from build123d import *

# Parameters (mm, degrees)
F1_DEPTH = 7.62
F3_DEPTH = 7.62


with BuildPart() as f1:
    # F0 (on Front) → F1 (new body)
    with BuildSketch(Plane.XZ):
        with BuildLine():
            ThreePointArc((21.0290110962, 0), (21.3248501657, 1.9931047456), (21.4237811773, 4.0056155995))
            ThreePointArc((21.4237811773, 4.0056155995), (-1.1080148506, 24.4259697619), (-19.2200190896, 0))
            ThreePointArc((-19.2200190896, 0), (0.9044960033, -16.5136695746), (21.0290110962, 0))
        make_face()
    extrude(amount=F1_DEPTH)

    # F2 (on Front) → F3 (join)
    with BuildSketch(Plane.XZ):
        with BuildLine():
            ThreePointArc((-16.8698355556, -6.6087017767), (-15.6905339278, -0.7832460117), (-21.5823259205, 0))
            ThreePointArc((-21.5823259205, 0), (-41.5234625412, -12.3382675542), (-47.9722805321, -34.8836556077))
            Line((-47.9722805321, -34.8836556077), (-35.7198044658, -33.9411571622))
            ThreePointArc((-35.7198044658, -33.9411571622), (-31.8794663631, -16.423449292), (-16.8698355556, -6.6087017767))
        make_face()
    extrude(amount=F3_DEPTH)


solid = f1.part
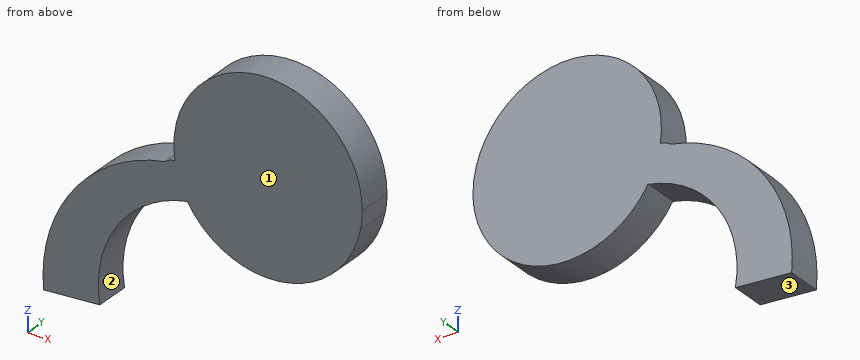
Geometry: final body of the model. Coordinates: model frame, mm. Face numbers are marked on the shaded views. Give positions to 0.01 mm unless a question says otherwise; leave off trailing zeros. Loops run counter-clockwise (first coordinate to the right, second up) from the corner with the lowest first, then second, coordinate; pieces in that order, holes last. Notation, with made-up numbers: (10, 31) -> (55, 31) arc R8 ccw to (55, 43) -> close; hole circle Ø3 at (11, 19.25). An arc over 180 degrees is marked (long way). Put each result on its own line as item: value.
1. Pull-direction query (X, two-part tool) for the marked faces 1, 2 and 3; classes: released by +X, released by -X, zero draft, split by the parting line, or undercut.
Taken from the geometry:
face 1: zero draft
face 2: undercut
face 3: released by +X
2. Ray query, line 1 along X through (y, z) = (-5, 4); line 2 along X through (y, z) = (-5.5, -19.5); line 3 along Z through (x, y) = (-13.5, -7). Return the intervals inside material, ascending. Write a range as [from, to].
Taken from the geometry:
line 1: x = [-19.61, 21.42]
line 2: x = [-45.63, -33.68]
line 3: z = [-10.61, 18.62]
3. Cut plane D-D (x = -24). Return the cut outline in (y, z).
Taken from the geometry:
outline: (-7.62, -9.23) -> (0, -9.23) -> (0, -0.55) -> (-7.62, -0.55) -> close
4. Pin query (flat end, axial travel): P1, Ø1, axis at x = -8, z = 11.5, coming from the +Y side; P2, Ø1.5, axis at x = 6.5, y = -4, coming from the -Z side; P3, Ø3, axis at y = -6.5, z = -23.5, coming from the +X side. Return the tip coordinate at first contact, or that it passes through.
Taken from the geometry:
P1: stops at y = 0
P2: stops at z = -15.93
P3: stops at x = -34.72
5. Cut plane C-C (z = 18). Return the cut outline in (x, y).
Taken from the geometry:
outline: (-14.1, -7.62) -> (15.91, -7.62) -> (15.91, 0) -> (-14.1, 0) -> close
6. Cut plane B-B (z = -10). Return the cut outline in (x, y), plus the area to 3 significant figures.
Taken from the geometry:
outline: (-39.58, -7.62) -> (-25.27, -7.62) -> (-25.27, 0) -> (-39.58, 0) -> close; (-14.09, -7.62) -> (15.9, -7.62) -> (15.9, 0) -> (-14.09, 0) -> close
area: 338 mm2
7. Cut plane A-A (y = -3.75). Return the cut outline in (x, z).
Taken from the geometry:
outline: (-47.97, -34.88) -> (-35.72, -33.94) arc R23.7 cw to (-16.87, -6.61) arc R4.07 ccw to (-16.72, -6.51) arc R20.52 ccw (long way) to (-19.38, 0.91) arc R4.07 ccw to (-21.58, 0) arc R32.5 ccw to start
